Read the model definition and answer for the solid it produces. Units are mm, in the model's axes. Face numbers are marked on the shaded views. A direction names the side the tool comes from. Give positions to 0.01 mm unless a question says otherwise; leave off trailing zeros. Order: outer loops, then holes, each group sorted by start corner. A loop starts at its lowest first (then second) coordinate and runs counter-clockwise, first axis right, second up. Notation, with made-up numbers: (7.25, 43) - (12.25, 43) arc R10 ccw to (12.25, 55) - close; hole circle Ø3 at (24.5, 74). An arc over 180 degrees is marked (long way). Return JSON: item names as keys, results as strings.
```python
from build123d import *

# Parameters (mm, degrees)
SKETCH_1_R      = 1
SKETCH_1_R_2    = 0.5
EXTRUDE_1_DEPTH = 2
FILLET_1_R      = 2
FILLET_2_R      = 2
EXTRUDE_START   = -3
SKETCH_3_R      = 1.1
SKETCH_3_R_2    = 0.5
SKETCH_3_R_3    = 2
SKETCH_3_R_4    = 1
EXTRUDE_3_DEPTH = 3


with BuildPart() as part:
    # 草图1 → 凸台-拉伸1 (new body)
    with BuildSketch(Plane.XY):
        Polygon((-10, -4), (10, -4), (2, 7), (2, 12), (0, 14), (-2, 12), (-2, 7), align=None)
        with Locations((-5, 0)):
            Circle(SKETCH_1_R, mode=Mode.SUBTRACT)
        with Locations((5, 0)):
            Circle(SKETCH_1_R, mode=Mode.SUBTRACT)
        with Locations((0, 12)):
            Circle(SKETCH_1_R_2, mode=Mode.SUBTRACT)
    extrude(amount=EXTRUDE_1_DEPTH)

    # 圆角1
    fillet_1_edges = [part.edges().sort_by_distance(p)[0] for p in [
        (0, 14, 1),
        (2, 12, 1),
        (-2, 12, 1),
        (-2, 7, 1),
        (2, 7, 1),
    ]]
    fillet(fillet_1_edges, radius=FILLET_1_R - 0.0001)  # a hair under: the kernel refuses the full size

    # 圆角2
    fillet_2_edges = [part.edges().sort_by_distance(p)[0] for p in [
        (10, -4, 1),
        (-10, -4, 1),
    ]]
    fillet(fillet_2_edges, radius=FILLET_2_R)

    # 草图3 → 凸台-拉伸3 (add)
    # profile 1 of 3: a face of its own
    with BuildSketch(Plane.XY.offset(2).offset(EXTRUDE_START)):
        with Locations((0, 12)):
            Circle(SKETCH_3_R)
        with Locations((0, 12)):
            Circle(SKETCH_3_R_2, mode=Mode.SUBTRACT)
    # profile 2 of 3: a face of its own
    with BuildSketch(Plane.XY.offset(2).offset(EXTRUDE_START)):
        with Locations((-5, 0)):
            Circle(SKETCH_3_R_3)
        with Locations((-5, 0)):
            Circle(SKETCH_3_R_4, mode=Mode.SUBTRACT)
    # profile 3 of 3: a face of its own
    with BuildSketch(Plane.XY.offset(2).offset(EXTRUDE_START)):
        with Locations((5, 0)):
            Circle(SKETCH_3_R_3)
        with Locations((5, 0)):
            Circle(SKETCH_3_R_4, mode=Mode.SUBTRACT)
    extrude(amount=EXTRUDE_3_DEPTH)


solid = part.part
```
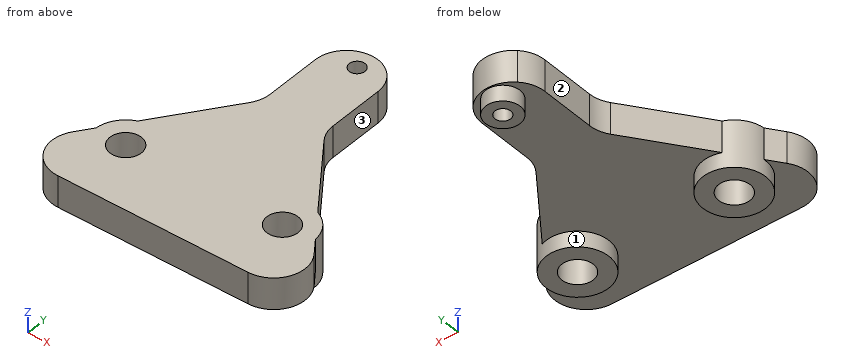
Q1. A cutting plane is placed at B-B (x = 0). Write down the section's boundary in (y, z), and give its area (3 significant figures).
Values:
{"outline": "(-4, 0) - (10.9, 0) - (10.9, -1) - (11.5, -1) - (11.5, 2) - (-4, 2) - close; (12.5, -1) - (13.1, -1) - (13.1, 0) - (13.17, 0) - (13.17, 2) - (12.5, 2) - close", "area": "33.5 mm²"}
Q2. For the marked faces 1, 2 and 3, determine the directions among +Z, -Z, +X, -X, +Y, -Y from which every point of the face is accessible in a straight line to the end or side of a thin tool.
Values:
{"face 1": "-Z", "face 2": "+Z, -Z, -X, +Y", "face 3": "+Z, -Z, +X, +Y"}
Q3. A cutting plane is placed at D-D (y = 12). Write down the section's boundary in (x, z), and give its area (3 significant figures).
Values:
{"outline": "(-1.82, 0) - (-1.1, 0) - (-1.1, -1) - (-0.5, -1) - (-0.5, 2) - (-1.82, 2) - close; (0.5, -1) - (1.1, -1) - (1.1, 0) - (1.82, 0) - (1.82, 2) - (0.5, 2) - close", "area": "6.48 mm²"}
Q4. A cutting plane is placed at A-A (z = -0.25). Write down the section's boundary in (x, y), and give its area (3 significant figures).
Values:
{"outline": "circle Ø4 at (-5, 0); circle Ø2.2 at (0, 12); circle Ø4 at (5, 0); hole circle Ø2 at (-5, 0); hole circle Ø1 at (0, 12); hole circle Ø2 at (5, 0)", "area": "21.9 mm²"}
Q5. A cutting plane is placed at C-C (z = 1.7). Give the number of separate pieces and of enclosed holes in the cut face, and give its area (3 significant figures).
Values:
{"separate pieces": "1", "enclosed holes": "3", "area": "142 mm²"}
Q6. Given pin 1 (1.8 mm diameter, centred on x = -5, y = 0, fed in from -Z); pin 2 (5 mm diameter, centred on x = -1, y = 6.5, fed in from -Z); pin 3 (1 mm diameter, centred on y = 2, z = 0, fed in from -X); pin 4 (1.6 mm diameter, centred on y = 8.5, z = 1, fed in from +X), each flat-ended and moving along its own axis, determine where each tip first touches the part or whether it passes through.
Values:
{"pin 1": "passes through", "pin 2": "stops at z = 0", "pin 3": "stops at x = -6.32", "pin 4": "stops at x = 2"}
Q7. Consider L1, parallel to X at y = -0.25, z = -0.6; L2, parallel to Z at x = 1.5, y = 1.25; L3, parallel to Y at x = 0, z = 1.25. Determine where each line is inside the solid, lowest interval first.
Values:
{"L1": "x = -6.98 to -5.97, -4.03 to -3.02, 3.02 to 4.03, 5.97 to 6.98", "L2": "z = 0 to 2", "L3": "y = -4 to 11.5, 12.5 to 13.17"}
